Work out the finished part from the listing and answer in its coordinate system (mm). A direction names the side the tool comes from. Round coordinates to 2 decimals unless told otherwise and drop trailing zeros. Write each loop counter-clockwise with the first axis right and the second up, starting at its lowest first coordinate (ties: lowest second). Pieces come first, ordered by that corner, then holes. Notation, with made-up numbers: M -16,23 L 2,23 A8 ccw 2,27 Z; hole C -5.75,-32.75 d1. An arc over 180 degrees is marked long. One line per item, written item: value. Start each with the question number.
Q1. Find section C-C (x = 3.5). Write down the section's boundary in (y, z).
Q2. The mould has two halves that part along Y. Classify faces 3 (the cylindrical face through (0.99, 9.15, 15.07)), 4 (the cylindrical face through (8.496, 0.986, 13.426)), 5 (the flat face through (9.3, 0, 77.4)): released by +Y, released by -Y, zero draft, split by the parting line, or undercut.
Q3. Given pin 1 Ø2 at (y, z) = (5.5, 105.5) entering from +X; pin 2 Ø1.5 at (x, z) = (4.5, 110.5) entering from +Y, each flat-ended and moving along its own axis, determine where each tip first touches the part or whether it passes through.
Q4. Find section A-A (z = 15). Write down the section's boundary in (x, y).
Q5. Find section B-B (z = 100). Write down the section's boundary in (x, y), and give its area (3 significant figures).
Q6. Consider probe 1 along Z at (x, y) = (0.4, 7.5); probe 2 along Y at (x, z) = (1.05, 79.5). Determine where each line is inside the solid, lowest interval first.
Q7. A tool of negligible diameter and unlimited length cuts with its end or side. For faces 1 (the cylindrical face through (0.99, 9.15, 79.57)), 2 (the flat face through (10, 2, 77)), from which of +Z, -Z, +X, -X, +Y, -Y can it reach the whole face along a straight path? Write none if from no direction.
from build123d import *

# Parameters (mm, degrees)
EXTRUDE_1_DEPTH          = 155
M4X0_7_1_D               = 3.3
M4X0_7_1_DEPTH           = 11.5
M4X0_7_1_TIP             = 0.991420021
M4X0_7_1_ON_FACE_2_D     = 3.3
M4X0_7_1_ON_FACE_2_DEPTH = 11.5
M4X0_7_1_ON_FACE_2_TIP   = 0.991420021
SKETCH_6_W               = 24.634949406
SKETCH_6_H               = 34.337648086
CUT_EXTRUDE_2_DEPTH      = 2


with BuildPart() as part:
    # ｽｹｯﾁ1 → ﾎﾞｽ - 押し出し1 (new body)
    with BuildSketch(Plane.XY):
        Polygon((0, 0), (0, 15), (2, 15), (2, 2), (15, 2), (15, 0), align=None)
    extrude(amount=EXTRUDE_1_DEPTH)

    # M4x0.7 ねじ穴1
    with Locations(Plane(origin=(2, 7.5, 140), x_dir=(0, 1, 0), z_dir=(1, 0, 0))):
        with Locations((0, 0), (0, -60.5), (0, -125)):
            Hole(M4X0_7_1_D / 2, depth=M4X0_7_1_DEPTH)
            with Locations((0, 0, -(M4X0_7_1_DEPTH + M4X0_7_1_TIP / 2))):  # 118° drill point
                Cone(0, M4X0_7_1_D / 2, M4X0_7_1_TIP, mode=Mode.SUBTRACT)

    # M4x0.7 ねじ穴1 on face 2
    with Locations(Plane(origin=(7.5, 2, 140), x_dir=(0, 0, 1), z_dir=(0, 1, 0))):
        with Locations((0, 0), (-62.5, 0), (-125, 0.5)):
            Hole(M4X0_7_1_ON_FACE_2_D / 2, depth=M4X0_7_1_ON_FACE_2_DEPTH)
            with Locations((0, 0, -(M4X0_7_1_ON_FACE_2_DEPTH + M4X0_7_1_ON_FACE_2_TIP / 2))):  # 118° drill point
                Cone(0, M4X0_7_1_ON_FACE_2_D / 2, M4X0_7_1_ON_FACE_2_TIP, mode=Mode.SUBTRACT)

    # ｽｹｯﾁ6 → ｶｯﾄ - 押し出し2 (cut)
    with BuildSketch(Plane(origin=(0, 0, 0), x_dir=(-1, 0, 0), z_dir=(0, 0, -1))):
        with Locations((-5.917994617, 11.841361704)):
            Rectangle(SKETCH_6_W, SKETCH_6_H)
    extrude(amount=-CUT_EXTRUDE_2_DEPTH, mode=Mode.SUBTRACT)


solid = part.part
The answers:
1. outline: M 0,2 L 2,2 L 2,155 L 0,155 Z
2. face 3: undercut
2. face 4: zero draft
2. face 5: released by -Y
3. pin 1: x = 2
3. pin 2: y = 2
4. outline: M 0,0 L 6.35,0 L 6.35,2 L 2,2 L 2,5.85 L 0,5.85 Z; M 0,9.15 L 2,9.15 L 2,15 L 0,15 Z; M 9.65,0 L 15,0 L 15,2 L 9.65,2 Z
5. outline: M 0,0 L 15,0 L 15,2 L 2,2 L 2,15 L 0,15 Z
5. area: 56.0 mm2
6. probe 1: 2 to 13.35, 16.65 to 77.85, 81.15 to 138.35, 141.65 to 155
6. probe 2: 0 to 5.85, 9.15 to 15
7. face 1: +X, -X
7. face 2: +Z, -Z, +X, +Y
